Here's how the part is built. I have some questions about the finished solid (model axes, mm). A direction names the side the tool comes from. Coordinates: 2 decimals unless noted, no trailing zeros. Write each loop counter-clockwise with the first axis right and the second up, starting at its lowest first coordinate (ties: lowest second). Pieces come first, ordered by that corner, then holes.
Item 1: If we section it at B-B (x = 0): Please give me the cut outline in (y, z), then the cut area to 4 significant figures.
Item 2: If we section it at C-C (y = 5.75): Please give me the cut outline in (x, z), then the cut area to 3 significant figures.
Item 3: If I drill on line 1 (Z direction, x = 0, y = 12.25); line 2 (X direction, y = 14.25, z = 0), over which ranges is the centre line in solid material (lowest first)?
Item 4: I'm going to push flat-ended pins straight in: pin 1 Ø4 at (x, z) = (-0.5, 3) entering from -Y; pin 2 Ø0.8 at (x, z) = (0, 0) entering from -Y; pin 3 Ø1 at (x, z) = (4, -1.5) entering from +Y; pin 4 Ø3 at (x, y) = (-2.5, 6.5) entering from +Z. Where does each tip first touch, or does it pass through?
Item 5: If we section it at A-A (y = 1.25): Please give me the cut outline in (x, z), then the cut area to 3 significant figures.
Item 6: If we section it at D-D (y = 13.25): Please give me the cut outline in (x, z).
Item 7: For faces 1 (the face through (0, 7, 0)), 2 (the face through (-1.08, 6.41, 4.88)), 3 (the face through (0, 13, 1)), which set-ups out of +Z, -Z, +X, -X, +Y, -Y let a thin tool reach every point of the face, with its end or its side?
Item 8: We'd pull the mould along Z, two halves only. Please class faces 4 (the face through (-0.465, 15.854, 2.095)), 5 (the face through (-0.03, 5.49, -2.76)), 6 (the face through (1, 16, 1)): +Z half, -Z half, draft (parallel to the pull), parting line (faces both ways), or undercut.
from build123d import *

# Parameters (mm, degrees)
SKETCH1_R           = 5
BOSS_EXTRUDE1_DEPTH = 16
CHAMFER1_SIZE       = 3
SKETCH2_R           = 1
CUT_EXTRUDE1_DEPTH  = 7
CUT_EXTRUDE2_DEPTH  = 7
CHAMFER2_SIZE       = 2.5


with BuildPart() as part:
    # Sketch1 → Boss-Extrude1 (new body)
    with BuildSketch(Plane(origin=(0, 0, 0), x_dir=(1, 0, 0), z_dir=(0, 1, 0))):
        Circle(SKETCH1_R)
    extrude(amount=BOSS_EXTRUDE1_DEPTH)

    # Chamfer1
    chamfer1_edges = [part.edges().sort_by_distance(p)[0] for p in [
        (-5, 16, 0),
    ]]
    chamfer(chamfer1_edges, length=CHAMFER1_SIZE)

    # Sketch2 → Cut-Extrude1 (cut)
    with BuildSketch(Plane(origin=(0, 16, 0), x_dir=(1, 0, 0), z_dir=(0, 1, 0))):
        Circle(SKETCH2_R)
    extrude(amount=-CUT_EXTRUDE1_DEPTH, mode=Mode.SUBTRACT)

    # Sketch3 → Cut-Extrude2 (cut)
    with BuildSketch(Plane.XZ):
        Polygon((-2.165063509, 3.75), (-4.330127019, 0), (-2.165063509, -3.75), (2.165063509, -3.75), (4.330127019, 0), (2.165063509, 3.75), align=None)
    extrude(amount=-CUT_EXTRUDE2_DEPTH, mode=Mode.SUBTRACT)

    # Chamfer2
    chamfer2_edges = [part.edges().sort_by_distance(p)[0] for p in [
        (0, 7, 3.75),
        (3.247595264, 7, 1.875),
        (3.247595264, 7, -1.875),
        (0, 7, -3.75),
        (-3.247595264, 7, -1.875),
        (-3.247595264, 7, 1.875),
    ]]
    chamfer(chamfer2_edges, length=CHAMFER2_SIZE)


solid = part.part
Answer list:
1. outline: (0, -5) - (13, -5) - (16, -2) - (16, -1) - (9, -1) - (9, 1) - (16, 1) - (16, 2) - (13, 5) - (0, 5) - (0, 3.75) - (4.5, 3.75) - (7, 1.25) - (7, -1.25) - (4.5, -3.75) - (0, -3.75) - close
1. area: 90.75 mm2
2. outline: circle Ø10 at (0, 0); hole (-2.89, 0) - (-1.44, -2.5) - (1.44, -2.5) - (2.89, 0) - (1.44, 2.5) - (-1.44, 2.5) - close
2. area: 56.9 mm2
3. line 1: z = -5 to -1, 1 to 5
3. line 2: x = -3.75 to -1, 1 to 3.75
4. pin 1: stops at y = 0
4. pin 2: stops at y = 7
4. pin 3: stops at y = 14.23
4. pin 4: stops at z = 4.9
5. outline: circle Ø10 at (0, 0); hole (-4.33, 0) - (-2.17, -3.75) - (2.17, -3.75) - (4.33, 0) - (2.17, 3.75) - (-2.17, 3.75) - close
5. area: 29.8 mm2
6. outline: circle Ø9.5 at (0, 0); hole circle Ø2 at (0, 0)
7. face 1: -Y
7. face 2: +Y, -Y
7. face 3: +Y
8. face 4: parting line
8. face 5: undercut
8. face 6: draft
